```python
from build123d import *

# Parameters (mm, degrees)
SKETCH1_R           = 3.556
BOSS_EXTRUDE1_DEPTH = 4.445


with BuildPart() as part:
    # Sketch1 → Boss-Extrude1 (new body)
    with BuildSketch(Plane(origin=(0, 0, 0), x_dir=(0, 0, -1), z_dir=(1, 0, 0))):
        with BuildLine():
            Line((-38.1, 47.288805643), (38.1, 47.288805643))
            ThreePointArc((38.1, 47.288805643), (46.5280051, 41.760994289), (44.815753872, 31.828413352))
            Line((44.815753872, 31.828413352), (8.061763365, -7.528573627))
            ThreePointArc((8.061763365, -7.528573627), (0, -11.030478204), (-8.061763365, -7.528573627))
            Line((-8.061763365, -7.528573627), (-44.815753872, 31.828413352))
            ThreePointArc((-44.815753872, 31.828413352), (-46.5280051, 41.760994289), (-38.1, 47.288805643))
        make_face()
        with Locations((-38.1, 38.1)):
            Circle(SKETCH1_R, mode=Mode.SUBTRACT)
        Circle(SKETCH1_R, mode=Mode.SUBTRACT)
        with Locations((38.1, 38.1)):
            Circle(SKETCH1_R, mode=Mode.SUBTRACT)
    extrude(amount=BOSS_EXTRUDE1_DEPTH)


solid = part.part
```
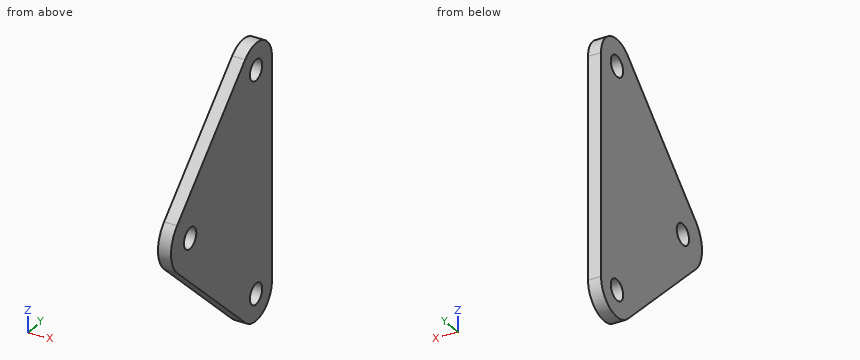
Can you work these out from the model? Positions are in its coordinate system, mm. Coordinates: 2 decimals unless noted, no trailing zeros. Loops run counter-clockwise (first coordinate to the right, second up) from the corner with the lowest first, then second, coordinate; pieces in that order, holes last. Notation, with made-up numbers: M -34.75,65 L -21.75,65 A11 cw -21.75,86 Z; hole C 28.5,-7 d11. An arc over 180 degrees is marked long. Put each result on its own line as item: value. Start each with the question number.
(1) Imagine slicing it at D-D on z = -2.5. List the corners of the cut face in (x, y) for me (3 decimals).
(2) Will these pins go through, and if not, where does the flat tip stop? pin 1 Ø4.5 at (y, z) = (38.1, -38.1) entering from +X; pin 2 Ø1.5 at (x, z) = (3, 20) entering from -Y.
(3) Imagine slicing it at B-B on x = 2.55. List the corners of the cut face in (y, z) for me.
(4) I need wall thicknesses on probe 1 along Y at (x, z) = (2.2, 37); probe 2 along Y at (x, z) = (2, -38.1); probe 3 along Z at (x, y) = (1.7, 12). Which ranges of each line are inside material? Lowest first, please.
(5) Imagine slicing it at C-C on y = -1. List the corners of the cut face in (x, z) for me (1 decimal).
(6) Imagine slicing it at A-A on y = 38.1. List the corners of the cut face in (x, z) for me (3 decimals), and give its area (3 significant figures).
Worked answers:
1. outline: M 0,-10.743 L 4.445,-10.743 L 4.445,-2.529 L 0,-2.529 Z; M 0,2.529 L 4.445,2.529 L 4.445,47.289 L 0,47.289 Z
2. pin 1: passes through
2. pin 2: stops at y = 4.45
3. outline: M -7.53,-8.06 L 31.83,-44.82 A9.19 ccw 47.29,-38.1 L 47.29,38.1 A9.19 ccw 31.83,44.82 L -7.53,8.06 A11.03 ccw Z; hole C 0,0 d7.11; hole C 38.1,-38.1 d7.11; hole C 38.1,38.1 d7.11
4. probe 1: y = 23.46 to 34.72, 41.48 to 47.29
4. probe 2: y = 24.64 to 34.54, 41.66 to 47.29
4. probe 3: z = -26.3 to 26.3
5. outline: M 0,-14.2 L 4.4,-14.2 L 4.4,-3.4 L 0,-3.4 Z; M 0,3.4 L 4.4,3.4 L 4.4,14.2 L 0,14.2 Z
6. outline: M 0,-47.289 L 4.445,-47.289 L 4.445,-41.656 L 0,-41.656 Z; M 0,-34.544 L 4.445,-34.544 L 4.445,34.544 L 0,34.544 Z; M 0,41.656 L 4.445,41.656 L 4.445,47.289 L 0,47.289 Z
6. area: 357 mm2
